Source: CAD feature listing. Evaluate the final solid. Frame: model axes, mm. Face numbers are marked on the shaded views. Coordinates: 2 decimals unless noted, no trailing zeros. Order: outer loops, then holes, each group sorted by start corner. A loop starts at its lowest first (then second) coordinate and runs counter-clockwise, first axis right, second up.
Item 1: Section A-A on z = 6.5. Return the cut outline in (x, y).
Item 2: Ray query, line 1 (Z direction, x = -2.5, y = 5.25); line 2 (X direction, y = -1.5, z = -12.5); line 3 (Z direction, x = -14.5, y = -2.5). Return the intervals inside material, ascending.
Item 3: Contact query for flat-ended pins moving along their axis: P1, Ø14.5, axis at x = -37, z = -9, coming from the -Y side; P2, Ø3, axis at x = 9.5, y = 1, coming from the +Z side; P3, Ø0.7, axis at x = -4.5, y = -6, coming from the +Z side; P4, Ø6, axis at x = -0.52, z = 39.1, coming from the +Y side. Output: stop coordinate, or through.
Item 4: Section B-B on x = 31. Return the cut outline in (y, z).
Item 5: Mould query, pull axis Z, two halves, no side actions, for the marked faces 1, 2 and 3. Classes: released by +Z, released by -Z, zero draft, split by the parting line, or undercut.
from build123d import *

# Parameters (mm, degrees)
SKETCH1_R               = 3.65
SKETCH1_W               = 26.6
SKETCH1_H               = 32.6
BOSS_EXTRUDE1_DEPTH     = 8
SKETCH2_W               = 3
SKETCH2_H               = 0.7
BOSS_EXTRUDE2_DEPTH     = 1.2
SKETCH3_W               = 3
SKETCH3_H               = 0.7
BOSS_EXTRUDE3_DEPTH     = 1.2
CHAMFER1_SIZE           = 1.2
CUT_EXTRUDE1_DEPTH      = 85.649459397
CUT_EXTRUDE1_DEPTH_BACK = 85.649459397
SKETCH4_W               = 48.801078557
SKETCH4_H               = 1.4
SKETCH4_W_2             = 10.59579159
SKETCH4_W_3             = 46.838011079
BOSS_EXTRUDE4_START     = -5.4
SKETCH5_W               = 13
SKETCH5_H               = 1.2
SKETCH5_W_2             = 1.2
SKETCH5_H_2             = 13
BOSS_EXTRUDE4_DEPTH     = 2.8
BOSS_EXTRUDE5_REACH     = 77.99
SKETCH7_W               = 1.2
SKETCH7_H               = 1.202104206
SKETCH7_H_2             = 1.201731925
BOSS_EXTRUDE6_DEPTH     = 7
SKETCH8_W               = 1.202104206
SKETCH8_H               = 1.3
SKETCH8_W_2             = 1.201731925
BOSS_EXTRUDE7_DEPTH     = 26.6
SKETCH9_W               = 1.2
SKETCH9_H               = 1.3
BOSS_EXTRUDE8_DEPTH     = 11.797895795


with BuildPart() as part:
    # Sketch1 → Boss-Extrude1 (new body)
    with BuildSketch(Plane(origin=(0, 0, 0), x_dir=(1, 0, 0), z_dir=(0, 1, 0))):
        with BuildLine():
            Line((-7.021942446, 23.451798561), (-15.021942446, 23.451798561))
            Line((-15.021942446, 23.451798561), (-15.021942446, 12.601798561))
            Line((-15.021942446, 12.601798561), (-45.721942446, 10.951798561))
            ThreePointArc((-45.721942446, 10.951798561), (-50.571942446, 6.101798561), (-45.721942446, 1.251798561))
            Line((-45.721942446, 1.251798561), (-15.021942446, -0.398201439))
            Line((-15.021942446, -0.398201439), (-15.021942446, -11.548201439))
            Line((-15.021942446, -11.548201439), (-7.021942446, -11.548201439))
            Line((-7.021942446, -11.548201439), (-5.371942446, -39.398201439))
            ThreePointArc((-5.371942446, -39.398201439), (-0.37187086, -43.955153005), (4.337327046, -39.098201439))
            Line((4.337327046, -39.098201439), (5.978057554, -11.548201439))
            Line((5.978057554, -11.548201439), (13.978057554, -11.548201439))
            Line((13.978057554, -11.548201439), (13.978057554, -0.398201439))
            Line((13.978057554, -0.398201439), (44.678057554, 1.251798561))
            ThreePointArc((44.678057554, 1.251798561), (49.528057554, 6.101798561), (44.678057554, 10.951798561))
            Line((44.678057554, 10.951798561), (13.978057554, 12.601798561))
            Line((13.978057554, 12.601798561), (13.978057554, 23.451798561))
            Line((13.978057554, 23.451798561), (5.978057554, 23.451798561))
            Line((5.978057554, 23.451798561), (4.328057554, 51.301798561))
            ThreePointArc((4.328057554, 51.301798561), (-0.521942446, 56.151798561), (-5.371942446, 51.301798561))
            Line((-5.371942446, 51.301798561), (-7.021942446, 23.451798561))
        make_face()
        with Locations(Location((-0.521942446, -39.098201439, 0), (0, 0, 270))):
            Circle(SKETCH1_R, mode=Mode.SUBTRACT)
        with BuildLine():
            Line((4.775953349, -11.548201439), (3.309960917, -36.110055423))
            ThreePointArc((3.309960917, -36.110055423), (-0.521942446, -34.238931946), (-4.35384581, -36.110055423))
            Line((-4.35384581, -36.110055423), (-5.819838241, -11.548201439))
            Line((-5.819838241, -11.548201439), (4.775953349, -11.548201439))
        make_face(mode=Mode.SUBTRACT)
        with Locations((-0.521942446, 5.951798561)):
            Rectangle(SKETCH1_W, SKETCH1_H, mode=Mode.SUBTRACT)
        with Locations(Location((-45.721942446, 6.101798561, 0), (0, 0, 270))):
            Circle(SKETCH1_R, mode=Mode.SUBTRACT)
        with BuildLine():
            Line((-42.720356894, 9.911389638), (-15.021942446, 11.400066636))
            Line((-15.021942446, 11.400066636), (-15.021942446, 0.803530486))
            Line((-15.021942446, 0.803530486), (-42.720356894, 2.292207484))
            ThreePointArc((-42.720356894, 2.292207484), (-40.871942446, 6.101798561), (-42.720356894, 9.911389638))
        make_face(mode=Mode.SUBTRACT)
        with BuildLine():
            Line((-5.819838241, 23.451798561), (-4.34653611, 48.319352702))
            ThreePointArc((-4.34653611, 48.319352702), (-0.521942446, 46.451798561), (3.302651218, 48.319352702))
            Line((3.302651218, 48.319352702), (4.775953349, 23.451798561))
            Line((4.775953349, 23.451798561), (-5.819838241, 23.451798561))
        make_face(mode=Mode.SUBTRACT)
        with Locations(Location((-0.521942446, 51.301798561, 0), (0, 0, 270))):
            Circle(SKETCH1_R, mode=Mode.SUBTRACT)
        with BuildLine():
            Line((41.676472002, 2.292207484), (13.978057554, 0.803530486))
            Line((13.978057554, 0.803530486), (13.978057554, 11.400066636))
            Line((13.978057554, 11.400066636), (41.676472002, 9.911389638))
            ThreePointArc((41.676472002, 9.911389638), (39.828057554, 6.101798561), (41.676472002, 2.292207484))
        make_face(mode=Mode.SUBTRACT)
        with Locations(Location((44.678057554, 6.101798561, 0), (0, 0, 270))):
            Circle(SKETCH1_R, mode=Mode.SUBTRACT)
    extrude(amount=BOSS_EXTRUDE1_DEPTH)

    # Sketch2 → Boss-Extrude2 (add)
    with BuildSketch(Plane.XY.offset(-22.251798561)):
        with Locations((-2.021942446, 6.05)):
            Rectangle(SKETCH2_W, SKETCH2_H)
        with Locations((0.978057554, 6.05)):
            Rectangle(SKETCH2_W, SKETCH2_H)
    extrude(amount=BOSS_EXTRUDE2_DEPTH)

    # Sketch3 → Boss-Extrude3 (add)
    with BuildSketch(Plane(origin=(0, 0, 10.348201439), x_dir=(-1, 0, 0), z_dir=(0, 0, -1))):
        with Locations((-0.978057554, 6.05)):
            Rectangle(SKETCH3_W, SKETCH3_H)
        with Locations((2.021942446, 6.05)):
            Rectangle(SKETCH3_W, SKETCH3_H)
    extrude(amount=BOSS_EXTRUDE3_DEPTH)

    # Chamfer1
    chamfer1_edges = [part.edges().sort_by_distance(p)[0] for p in [
        (-0.521942446, 5.7, -22.251798561),
        (-0.521942446, 5.7, 10.348201439),
    ]]
    chamfer(chamfer1_edges, length=CHAMFER1_SIZE - 0.0001)  # a hair under: the kernel refuses the full size

    # Sketch4 → Cut-Extrude1 (cut, two sides: drawn at the far end of the back side and taken through both)
    with BuildSketch(Plane(origin=(0, 0, -23.451798561), x_dir=(-1, 0, 0), z_dir=(0, 0, -1)).offset(-CUT_EXTRUDE1_DEPTH_BACK)):
        with Locations((-29.176492628, 3.3)):
            Rectangle(SKETCH4_W, SKETCH4_H)
        with Locations((-29.176492628, 4.7)):
            Rectangle(SKETCH4_W, SKETCH4_H)
        with Locations((0.521942446, 4.7)):
            Rectangle(SKETCH4_W_2, SKETCH4_H)
        with Locations((0.521942446, 3.3)):
            Rectangle(SKETCH4_W_2, SKETCH4_H)
        with Locations((29.238843781, 3.3)):
            Rectangle(SKETCH4_W_3, SKETCH4_H)
        with Locations((29.238843781, 4.7)):
            Rectangle(SKETCH4_W_3, SKETCH4_H)
    extrude(amount=CUT_EXTRUDE1_DEPTH + CUT_EXTRUDE1_DEPTH_BACK, mode=Mode.SUBTRACT)


with BuildPart() as cut_extrude1_piece_1:
    # of the separate pieces the step leaves, piece 1, a body of its own (cut_extrude1_pieces)
    add(part.part.solids().sort_by_distance((-3.521942446, 6.4, 10.348201439))[0])



with BuildPart() as cut_extrude1_piece_2:
    # of the separate pieces the step leaves, piece 2, a body of its own (cut_extrude1_pieces)
    add(part.part.solids().sort_by_distance((12.778057554, 2.6, 10.348201439))[0])


with BuildPart() as cut_extrude1_piece_1_1:
    add(cut_extrude1_piece_1.part)

    add(cut_extrude1_piece_2.part)  # Boss-Extrude4 merges Cut-Extrude1 piece 2
    # Sketch5 → Boss-Extrude4 (add)
    with BuildSketch(Plane(origin=(0, 8, 0), x_dir=(1, 0, 0), z_dir=(0, 1, 0)).offset(BOSS_EXTRUDE4_START)):
        with Locations((-0.521942446, 22.851798561)):
            Rectangle(SKETCH5_W, SKETCH5_H)
        with Locations((-0.521942446, -10.948201439)):
            Rectangle(SKETCH5_W, SKETCH5_H)
        with Locations((-14.421942446, 6.101798561)):
            Rectangle(SKETCH5_W_2, SKETCH5_H_2)
        with Locations((13.378057554, 6.101798561)):
            Rectangle(SKETCH5_W_2, SKETCH5_H_2)
    extrude(amount=BOSS_EXTRUDE4_DEPTH)

    # Sketch6 → Boss-Extrude5 (add, up to next)
    with BuildSketch(Plane(origin=(0, 8, 0), x_dir=(1, 0, 0), z_dir=(0, 1, 0)), mode=Mode.PRIVATE) as boss_extrude5_sk1:
        with BuildLine():
            Line((-5.371942446, 51.301798561), (-4.171942446, 51.301798561))
            ThreePointArc((-4.171942446, 51.301798561), (-0.521942446, 54.951798561), (3.128057554, 51.301798561))
            Line((3.128057554, 51.301798561), (4.328057554, 51.301798561))
            ThreePointArc((4.328057554, 51.301798561), (-0.521942446, 56.151798561), (-5.371942446, 51.301798561))
        make_face()
    boss_extrude5_tool1 = extrude(boss_extrude5_sk1.sketch, amount=-BOSS_EXTRUDE5_REACH, mode=Mode.PRIVATE) - cut_extrude1_piece_1_1.part
    # Sketch6 → Boss-Extrude5 (add, up to next)
    with BuildSketch(Plane(origin=(0, 8, 0), x_dir=(1, 0, 0), z_dir=(0, 1, 0)), mode=Mode.PRIVATE) as boss_extrude5_sk2:
        with BuildLine():
            Line((3.128057554, -39.098201439), (4.328057554, -39.098201439))
            ThreePointArc((4.328057554, -39.098201439), (-0.521942446, -43.948201439), (-5.371942446, -39.098201439))
            Line((-5.371942446, -39.098201439), (-4.171942446, -39.098201439))
            ThreePointArc((-4.171942446, -39.098201439), (-0.521942446, -42.748201439), (3.128057554, -39.098201439))
        make_face()
    boss_extrude5_tool2 = extrude(boss_extrude5_sk2.sketch, amount=-BOSS_EXTRUDE5_REACH, mode=Mode.PRIVATE) - cut_extrude1_piece_1_1.part
    # Sketch6 → Boss-Extrude5 (add, up to next)
    with BuildSketch(Plane(origin=(0, 8, 0), x_dir=(1, 0, 0), z_dir=(0, 1, 0)), mode=Mode.PRIVATE) as boss_extrude5_sk3:
        with BuildLine():
            Line((44.678057554, 9.751798561), (44.678057554, 10.951798561))
            ThreePointArc((44.678057554, 10.951798561), (49.528057554, 6.101798561), (44.678057554, 1.251798561))
            Line((44.678057554, 1.251798561), (44.678057554, 2.451798561))
            ThreePointArc((44.678057554, 2.451798561), (48.328057554, 6.101798561), (44.678057554, 9.751798561))
        make_face()
    boss_extrude5_tool3 = extrude(boss_extrude5_sk3.sketch, amount=-BOSS_EXTRUDE5_REACH, mode=Mode.PRIVATE) - cut_extrude1_piece_1_1.part
    # Sketch6 → Boss-Extrude5 (add, up to next)
    with BuildSketch(Plane(origin=(0, 8, 0), x_dir=(1, 0, 0), z_dir=(0, 1, 0)), mode=Mode.PRIVATE) as boss_extrude5_sk4:
        with BuildLine():
            Line((-45.721942446, 1.251798561), (-45.721942446, 2.451798561))
            ThreePointArc((-45.721942446, 2.451798561), (-49.371942446, 6.101798561), (-45.721942446, 9.751798561))
            Line((-45.721942446, 9.751798561), (-45.721942446, 10.951798561))
            ThreePointArc((-45.721942446, 10.951798561), (-50.571942446, 6.101798561), (-45.721942446, 1.251798561))
        make_face()
    boss_extrude5_tool4 = extrude(boss_extrude5_sk4.sketch, amount=-BOSS_EXTRUDE5_REACH, mode=Mode.PRIVATE) - cut_extrude1_piece_1_1.part
    add(boss_extrude5_tool1.solids().sort_by_distance((-4.771942, 8, -51.410248))[0])
    add(boss_extrude5_tool2.solids().sort_by_distance((-0.521942, 8, 43.839752))[0])
    add(boss_extrude5_tool3.solids().sort_by_distance((44.786507, 8, -10.351799))[0])
    add(boss_extrude5_tool4.solids().sort_by_distance((-45.830392, 8, -10.351799))[0])

    # Sketch7 → Boss-Extrude6 (add)
    with BuildSketch(Plane.XZ):
        with Locations((-14.421942446, -0.202850664)):
            Rectangle(SKETCH7_W, SKETCH7_H)
        with Locations((-14.421942446, -12.000932599)):
            Rectangle(SKETCH7_W, SKETCH7_H_2)
        with Locations((13.378057554, -0.202850664)):
            Rectangle(SKETCH7_W, SKETCH7_H)
        with Locations((13.378057554, -12.000932599)):
            Rectangle(SKETCH7_W, SKETCH7_H_2)
    extrude(amount=BOSS_EXTRUDE6_DEPTH)

    # Sketch8 → Boss-Extrude7 (add)
    with BuildSketch(Plane(origin=(-13.821942446, 0, 0), x_dir=(0, 0, -1), z_dir=(1, 0, 0))):
        with Locations((0.202850664, -6.35)):
            Rectangle(SKETCH8_W, SKETCH8_H)
        with Locations((12.000932599, -6.35)):
            Rectangle(SKETCH8_W_2, SKETCH8_H)
    extrude(amount=BOSS_EXTRUDE7_DEPTH)

    # Sketch9 → Boss-Extrude8 (add)
    with BuildSketch(Plane(origin=(0, 0, -12.601798561), x_dir=(-1, 0, 0), z_dir=(0, 0, -1))):
        with Locations((-13.378057554, -6.35)):
            Rectangle(SKETCH9_W, SKETCH9_H)
        with Locations((14.421942446, -6.35)):
            Rectangle(SKETCH9_W, SKETCH9_H)
    extrude(amount=-BOSS_EXTRUDE8_DEPTH)


solid = cut_extrude1_piece_1_1.part
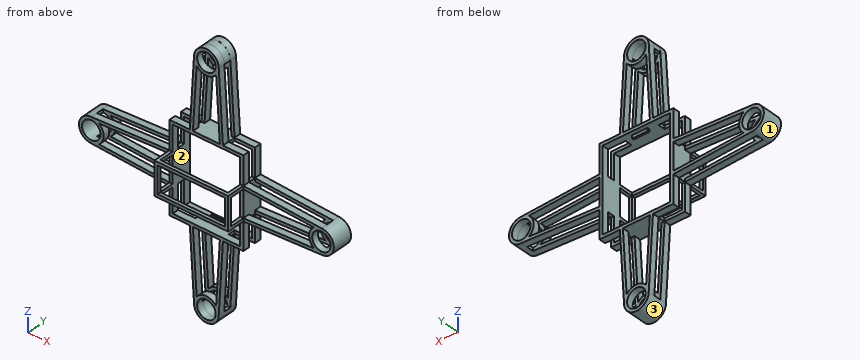
Answer list:
1. outline: (-15.02, 0) - (-13.82, 0) - (-13.82, 2.6) - (-15.02, 2.6) - close; (-15.02, 5.4) - (-13.82, 5.4) - (-13.82, 8) - (-15.02, 8) - close; (12.78, 0) - (13.98, 0) - (13.98, 2.6) - (12.78, 2.6) - close; (12.78, 5.4) - (13.98, 5.4) - (13.98, 8) - (12.78, 8) - close
2. line 1: z = -55.73 to -54.37, -23.45 to -22.25, 10.35 to 11.55, 42.17 to 43.53
2. line 2: x = -15.02 to -13.82, 12.78 to 13.98
2. line 3: z = -12.6 to -11.4, -0.8 to 0.4
3. P1: stops at y = 0
3. P2: stops at z = 11.55
3. P3: stops at z = 0.4
3. P4: passes through
4. outline: (0, -11.69) - (2.6, -11.69) - (2.6, -10.49) - (0, -10.49) - close; (0, -1.72) - (2.6, -1.72) - (2.6, -0.52) - (0, -0.52) - close; (5.4, -11.69) - (8, -11.69) - (8, -10.49) - (5.4, -10.49) - close; (5.4, -1.72) - (8, -1.72) - (8, -0.52) - (5.4, -0.52) - close
5. face 1: split by the parting line
5. face 2: undercut
5. face 3: released by -Z
